The listing builds one solid part. Answer for the finished solid, in the listing's coordinates (mm). A direction names the side the tool comes from. Round coordinates to 2 decimals unless told otherwise and drop trailing zeros. Write each loop counter-clockwise with the first axis right and the second up, starting at its lowest first coordinate (ties: lowest second). Pieces come first, ordered by that corner, then holes. Notation, with made-up numbers: (57.5, 16) - (68.5, 16) arc R23 cw to (68.5, 33) - close; hole circle Ø3 at (9, 21.25). An arc over 180 degrees is marked (long way). Return JSON: item names as keys, results as strings. Group by question number.
(1) Section C-C, the plane y = -6 is taken. Write down the section's boundary in (x, z), then the cut area to 3 significant figures.
(2) Section B-B, the plane x = 0 is taken. Write down the section's boundary in (y, z).
(3) Which of the six approach directions +Z, -Z, +X, -X, +Y, -Y give full straight-line access (tool end or side, diameter ignored) to faces 5 (the flat face through (-17.5, -16, 1)), 6 (the cylindrical face through (-0.54, 16.76, -37.56)), 7 (the flat face through (0, -16, 1))?
(4) Determine the mould class of faces 1 (the flat face through (-1, -17, -88)), 2 (the flat face through (0, 17.5, 1)), 3 (the flat face through (-16, -14, 1)), 4 (the flat face through (0, -17.5, 1)) for opening direction Y: +Y half, -Y half, draft (parallel to the pull), parting line (faces both ways), or undercut.
(5) Find the intervals of material crossed by line 1 along Z through (x, y) = (0, 16.5); line 2 along Y through (x, z) = (-13, -73.5), in increasing order. Write a range as [from, to].
(6) Section D-D, the plane x = -11.5 is taken. Write down the section's boundary in (y, z).
(7) Section A-A, the plane z = 19 is taken. Write down the section's boundary in (x, y).
```python
from build123d import *

# Parameters (mm, degrees)
MOTORBLOCKSKETCH_W         = 35
MOTORBLOCKSKETCH_H         = 35
MOTORBLOCKSKETCH_W_2       = 32
MOTORBLOCKSKETCH_H_2       = 32
BOSS_EXTRU_1_DEPTH         = 88
ESQUISSE3_W                = 80
ESQUISSE3_H                = 25
ENL_V_MAT_EXTRU_1_DEPTH    = 36
DRILLLEFTMOTORFIXSKETCH_R  = 2.5
ENL_V_MAT_EXTRU_2_DEPTH    = 5
DRILLRIGHTMOTORFIXSKETCH_R = 2.5
ENL_V_MAT_EXTRU_3_DEPTH    = 5


with BuildPart() as part:
    # MotorBlockSketch → Boss.-Extru.1 (new body, symmetric)
    with BuildSketch(Plane.XY):
        Rectangle(MOTORBLOCKSKETCH_W, MOTORBLOCKSKETCH_H)
        Rectangle(MOTORBLOCKSKETCH_W_2, MOTORBLOCKSKETCH_H_2, mode=Mode.SUBTRACT)
    extrude(amount=BOSS_EXTRU_1_DEPTH, both=True)

    # Esquisse3 → Enlèv. mat.-Extru.1 (cut, through all)
    with BuildSketch(Plane(origin=(17.5, 0, 0), x_dir=(0, 0, -1), z_dir=(1, 0, 0))):
        Rectangle(ESQUISSE3_W, ESQUISSE3_H)
    extrude(amount=-ENL_V_MAT_EXTRU_1_DEPTH, mode=Mode.SUBTRACT)

    # DrillLeftMotorFixSketch → Enlèv. mat.-Extru.2 (cut)
    with BuildSketch(Plane(origin=(0, 17.5, 0), x_dir=(1, 0, 0), z_dir=(0, 1, 0))):
        with Locations((0, 40)):
            Circle(DRILLLEFTMOTORFIXSKETCH_R)
    extrude(amount=-ENL_V_MAT_EXTRU_2_DEPTH, mode=Mode.SUBTRACT)

    # DrillRightMotorFixSketch → Enlèv. mat.-Extru.3 (cut)
    with BuildSketch(Plane(origin=(0, 17.5, 0), x_dir=(1, 0, 0), z_dir=(0, 1, 0))):
        with Locations((0, -40)):
            Circle(DRILLRIGHTMOTORFIXSKETCH_R)
    extrude(amount=-ENL_V_MAT_EXTRU_3_DEPTH, mode=Mode.SUBTRACT)


solid = part.part
```
Working result:
{
 "1": {"outline": "(-17.5, -88) - (-16, -88) - (-16, -40) - (-17.5, -40) - close; (-17.5, 40) - (-16, 40) - (-16, 88) - (-17.5, 88) - close; (16, -88) - (17.5, -88) - (17.5, -40) - (16, -40) - close; (16, 40) - (17.5, 40) - (17.5, 88) - (16, 88) - close", "area": "288 mm^2"},
 "2": {"outline": "(-17.5, -88) - (-16, -88) - (-16, 88) - (-17.5, 88) - close; (16, -88) - (17.5, -88) - (17.5, -42.5) - (16, -42.5) - close; (16, -37.5) - (17.5, -37.5) - (17.5, 37.5) - (16, 37.5) - close; (16, 42.5) - (17.5, 42.5) - (17.5, 88) - (16, 88) - close"},
 "3": {"face 5": "+Z, -Z, -X, +Y, -Y", "face 6": "+Y", "face 7": "+Z, -Z"},
 "4": {"face 1": "draft", "face 2": "+Y half", "face 3": "undercut", "face 4": "-Y half"},
 "5": {"line 1": "z = [-88, -42.5], [-37.5, 37.5], [42.5, 88]", "line 2": "y = [-17.5, -16], [16, 17.5]"},
 "6": {"outline": "(-17.5, -88) - (-16, -88) - (-16, 88) - (-17.5, 88) - close; (16, -88) - (17.5, -88) - (17.5, 88) - (16, 88) - close"},
 "7": {"outline": "(-17.5, -17.5) - (17.5, -17.5) - (17.5, -12.5) - (16, -12.5) - (16, -16) - (-16, -16) - (-16, -12.5) - (-17.5, -12.5) - close; (-17.5, 12.5) - (-16, 12.5) - (-16, 16) - (16, 16) - (16, 12.5) - (17.5, 12.5) - (17.5, 17.5) - (-17.5, 17.5) - close"}
}
